```python
from build123d import *

# Parameters (mm, degrees)
BOSS_EXTRUDE1_DEPTH = 40
SKETCH2_W           = 20
SKETCH2_H           = 42
CUT_EXTRUDE1_DEPTH  = 27
SKETCH3_R           = 15
CUT_EXTRUDE2_DEPTH  = 10


with BuildPart() as part:
    # Sketch1 → Boss-Extrude1 (new body)
    with BuildSketch(Plane.XY):
        with BuildLine():
            Line((0, 40), (70, 40))
            Line((70, 40), (70, -40))
            Line((70, -40), (0, -40))
            ThreePointArc((0, -40), (-40, 0), (0, 40))
        make_face()
    extrude(amount=BOSS_EXTRUDE1_DEPTH)

    # Sketch2 → Cut-Extrude1 (cut)
    with BuildSketch(Plane.XY.offset(40)):
        with Locations((60, -0.432961974)):
            Rectangle(SKETCH2_W, SKETCH2_H)
    extrude(amount=-CUT_EXTRUDE1_DEPTH, mode=Mode.SUBTRACT)

    # Sketch3 → Cut-Extrude2 (cut)
    with BuildSketch(Plane.XY.offset(40)):
        Circle(SKETCH3_R)
    extrude(amount=-CUT_EXTRUDE2_DEPTH, mode=Mode.SUBTRACT)


solid = part.part
```
The model under review builds one solid part; all positions refer to its coordinate system, in mm. A direction names the side the tool comes from. Give positions to 0.01 mm unless a question says otherwise; leave off trailing zeros. Write each loop counter-clockwise with the first axis right and the second up, starting at its lowest first coordinate (ties: lowest second). Pieces come first, ordered by that corner, then holes. Notation, with made-up numbers: M 54.25,51 L 63.25,51 A17 ccw 63.25,56 Z; hole C -27.75,38 d3. An arc over 180 degrees is marked long. Write item = value, one per line. Start each with the question number.
Q1. We need section A-A (y = 0). State the section outline as (x, z) points.
Q2. We need section C-C (z = 7). State the section outline as (x, y) points, plus the area to 3 significant figures.
Q3. We need section D-D (x = -28.5). State the section outline as (y, z) points.
Q4. Clearance check with flat-ended pins moving along their axes: pin 1 (12 mm diameter, centred on y = 4.5, z = 6, fed in from -X); pin 2 (1 mm diameter, centred on x = -5, z = 15, fed in from +Y); pin 3 (3 mm diameter, centred on x = -25.5, z = 33.5, fed in from +Y); pin 4 (3 mm diameter, centred on x = 34.5, y = 16, fed in from -Z). State where each tip first meets the part, or that it passes through.
Q5. Mouldability with a two-part tool opening along Y and no side actions: class faces 1 (the face through (35, -40, 20)), 2 (the face through (-39.99, -0.88, 19.72)), 3 (the face through (60, 20.567, 27)), 4 (the face through (70, 1, 11)) as released by +Y, released by -Y, zero draft, split by the parting line, or undercut.
Q6. For line 1 (Y direction, x = 0, z = 36); line 2 (Y direction, x = 64, z = 25); line 3 (Z direction, x = 13, y = -2.5), list the stretches that pass through material, from the lowest coordinate up.
Q7. Machinability: for faces 5 (the face through (60, -21.433, 27)), 6 (the face through (35, 40, 20)), 7 (the face through (-14.985, 0.66, 35.07)), which of the approach directions +Z, -Z, +X, -X, +Y, -Y give a long, thin tool a straight path to every point of the face, cutting with its end or side? Answer none if there is none.
Q8. We need section B-B (x = 8.5). State the section outline as (y, z) points.
Result set:
q1.outline = M -40,0 L 70,0 L 70,13 L 50,13 L 50,40 L 15,40 L 15,30 L -15,30 L -15,40 L -40,40 Z
q2.outline = M 0,-40 L 70,-40 L 70,40 L 0,40 A40 ccw Z
q2.area = 8,110 mm2
q3.outline = M -28.07,0 L 28.07,0 L 28.07,40 L -28.07,40 Z
q4.pin_1 = -40
q4.pin_2 = 39.75
q4.pin_3 = 32
q4.pin_4 = 0
q5.face_1 = released by -Y
q5.face_2 = split by the parting line
q5.face_3 = undercut
q5.face_4 = zero draft
q6.line_1 = -40 to -15, 15 to 40
q6.line_2 = -40 to -21.43, 20.57 to 40
q6.line_3 = 0 to 30
q7.face_5 = +Z, +X
q7.face_6 = +Z, -Z, +X, -X, +Y
q7.face_7 = +Z
q8.outline = M -40,0 L 40,0 L 40,40 L 12.36,40 L 12.36,30 L -12.36,30 L -12.36,40 L -40,40 Z
